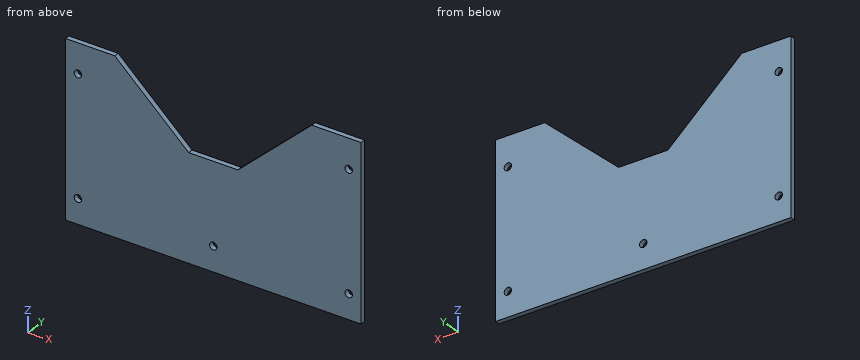
```python
from build123d import *

# Parameters (mm, degrees)
SKETCH1_R           = 1.905
BOSS_EXTRUDE1_DEPTH = 1.27


with BuildPart() as part:
    # Sketch1 → Boss-Extrude1 (new, symmetric)
    with BuildSketch(Plane(origin=(0, 0, 0), x_dir=(1, 0, 0), z_dir=(0, 1, 0))):
        Polygon((-76.2, 39.789919355), (76.2, 39.789919355), (76.2, -49.110080645), (50.8, -49.110080645), (12.7, -14.458198925), (-12.7, -14.458198925), (-50.8, -49.110080645), (-76.2, -49.110080645), align=None)
        with Locations(Location((69.85, 27.089919355, 0), (0, 0, 270))):
            Circle(SKETCH1_R, mode=Mode.SUBTRACT)
        with Locations(Location((0, 27.089919355, 0), (0, 0, 270))):
            Circle(SKETCH1_R, mode=Mode.SUBTRACT)
        with Locations(Location((-69.85, 27.089919355, 0), (0, 0, 270))):
            Circle(SKETCH1_R, mode=Mode.SUBTRACT)
        with Locations(Location((69.85, -33.870080645, 0), (0, 0, 270))):
            Circle(SKETCH1_R, mode=Mode.SUBTRACT)
        with Locations(Location((-69.85, -33.870080645, 0), (0, 0, 270))):
            Circle(SKETCH1_R, mode=Mode.SUBTRACT)
    extrude(amount=BOSS_EXTRUDE1_DEPTH, both=True)


solid = part.part
```
Read the model definition and answer for the solid it produces. Units are mm, in the model's axes. Give positions to 0.01 mm unless a question says otherwise; leave off trailing zeros. Order: outer loops, then holes, each group sorted by start corner. A loop starts at its lowest first (then second) coordinate and runs counter-clockwise, first axis right, second up.
(1) Find section D-D (z = 24). Give the vertices of the cut face in (x, y).
(2) Find section B-B (x = 0). Give the vertices of the cut face in (y, z), plus the area to 3 significant figures.
(3) Find section A-A (x = 69.85). Give the vertices of the cut face in (y, z).
(4) Find section C-C (y = 0.1). Give the vertices of the cut face in (x, z) (3 decimals), plus the area to 3 significant figures.
(5) Given pin 1 (1.5 mm diameter, centred on x = 17, y = -1, fed in from +Z); pin 2 (3 mm diameter, centred on x = 69.85, z = 33.87, fed in from -Y), each flat-ended and moving along its own axis, determine where each tip first touches the part or whether it passes through.
(6) Straight lines are drawn through the part: L1, parallel to X at y = 0.55, z = 33; L2, parallel to Z at x = 6.5, y = -0.9; L3, parallel to X at y = 0.25, z = 15. For each, find the intervals that lie inside material, in ascending order.
Result sheet:
1. outline: (-76.2, -1.27) - (-23.19, -1.27) - (-23.19, 1.27) - (-76.2, 1.27) - close; (23.19, -1.27) - (76.2, -1.27) - (76.2, 1.27) - (23.19, 1.27) - close
2. outline: (-1.27, -39.79) - (1.27, -39.79) - (1.27, -28.99) - (-1.27, -28.99) - close; (-1.27, -25.18) - (1.27, -25.18) - (1.27, 14.46) - (-1.27, 14.46) - close
2. area: 128 mm2
3. outline: (-1.27, -39.79) - (1.27, -39.79) - (1.27, -28.99) - (-1.27, -28.99) - close; (-1.27, -25.18) - (1.27, -25.18) - (1.27, 31.97) - (-1.27, 31.97) - close; (-1.27, 35.78) - (1.27, 35.78) - (1.27, 49.11) - (-1.27, 49.11) - close
4. outline: (-76.2, -39.79) - (76.2, -39.79) - (76.2, 49.11) - (50.8, 49.11) - (12.7, 14.458) - (-12.7, 14.458) - (-50.8, 49.11) - (-76.2, 49.11) - close; hole circle Ø3.81 at (-69.85, -27.09); hole circle Ø3.81 at (-69.85, 33.87); hole circle Ø3.81 at (0, -27.09); hole circle Ø3.81 at (69.85, -27.09); hole circle Ø3.81 at (69.85, 33.87)
4. area: 11,300 mm2
5. pin 1: stops at z = 19.05
5. pin 2: passes through
6. L1: x = -76.2 to -71.54, -68.16 to -33.09, 33.09 to 68.16, 71.54 to 76.2
6. L2: z = -39.79 to 14.46
6. L3: x = -76.2 to -13.3, 13.3 to 76.2
